Check sheet for the drawn part. Datum: minimum x, y, z corner. Units: mm. A direction names the side the tool comes from. Coordinates: 2 decimals unless noted, no trailing zeros. Write each loop counter-clockwise with the first axis right and the second up, starting at its lowest first coordinate (ties: lowest second). Pieces come first, ordered by that corner, then holes. Notation, with made-up numbers: M -0.75,61.5 L 53.25,61.5 A16 ccw 53.25,82.5 Z; hole C 61.5,60.25 d8. An arc over 180 degrees is marked long. Answer as CSV lines item,"result".
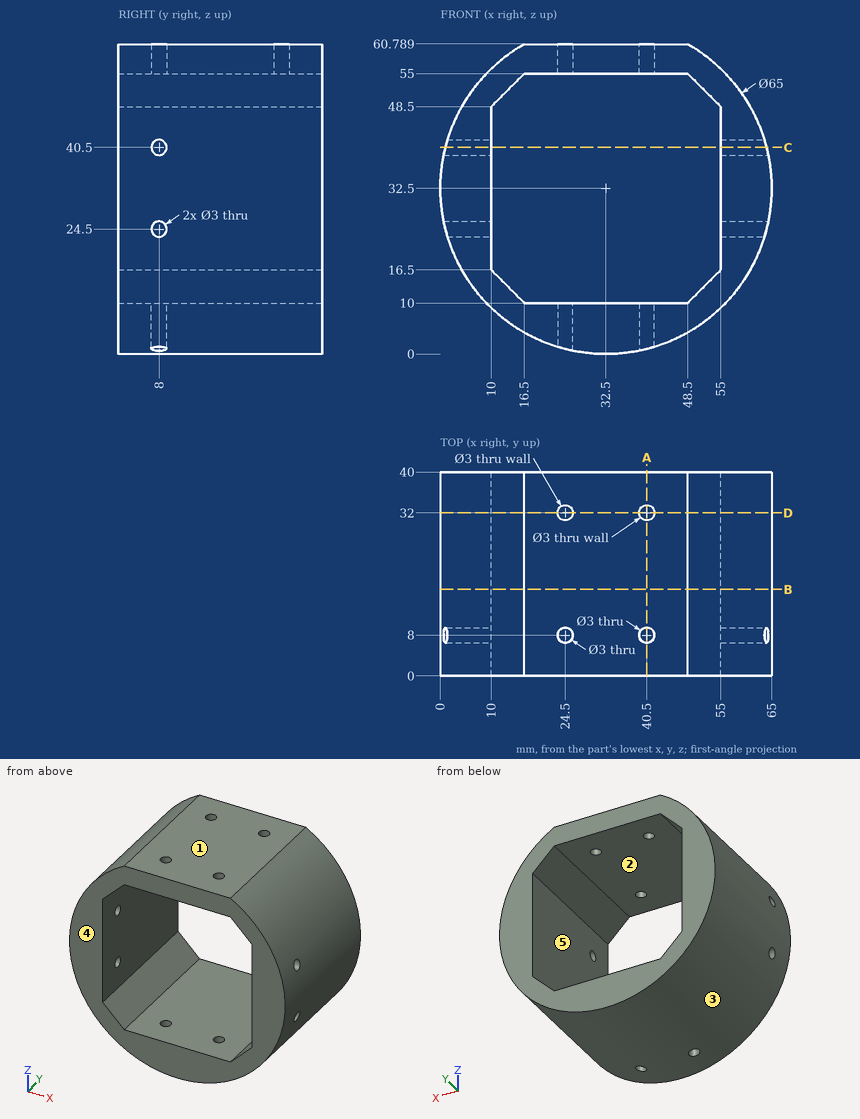
1) Section check C-C, the plane z = 40.5. Record the boundary of the cut face in (x, y), plus the area to 3 significant figures.
Answer key:
outline,"M 1,0 L 10,0 L 10,6.5 L 1,6.5 Z; M 1,9.5 L 10,9.5 L 10,40 L 1,40 Z; M 55,0 L 64,0 L 64,6.5 L 55,6.5 Z; M 55,9.5 L 64,9.5 L 64,40 L 55,40 Z"
area,"666 mm2"
2) Section check D-D, the plane y = 32. Record the boundary of the cut face in (x, z).
Answer key:
outline,"M 10,16.5 L 10,48.5 L 16.5,55 L 23,55 L 23,60.79 L 16.5,60.79 A32.5 ccw long 48.5,60.79 L 42,60.79 L 42,55 L 48.5,55 L 55,48.5 L 55,16.5 L 48.5,10 L 16.5,10 Z; M 26,55 L 39,55 L 39,60.79 L 26,60.79 Z"
3) Thickness scan on line 1 along Z through (x, y) = (41, 18); line 2 along Y through (x, z) = (5, 24) (1 decimal); line 3 along X through (y, z) = (4.5, 42.5). Record the ranges inside material, lowest first.
Answer key:
line 1,"z = 1.13 to 10, 55 to 60.79"
line 2,"y = 0 to 6.6, 9.4 to 40"
line 3,"x = 1.58 to 10, 55 to 63.42"
4) Depth check by flat-ended pin: P1, Ø1.5, axis at x = 52.5, y = 25, coming from the +Z side (1 decimal); P2, Ø4, axis at x = 24.5, y = 8, coming from the -Z side; P3, Ø16, axis at y = 19.5, z = 28.5, coming from the -X side; P4, Ø2.5, axis at y = 8, z = 24.5, coming from the -X side. Enter the tip coordinate at first touch or a pass-through.
Answer key:
P1,"stops at z = 58.7"
P2,"stops at z = 0.56"
P3,"stops at x = 0"
P4,"passes through"
5) Tool access check on the marked faces 4 and 5. Record the directions out of +Z, -Z, +X, -X, +Y, -Y that give a thin tool (end or side, any length) a straight path to the whole face; none if there is none.
Answer key:
face 4,"+Z, -Z, +X, -X, -Y"
face 5,"+Y, -Y"
6) Section check B-B, the plane y = 17. Record the boundary of the cut face in (x, z).
Answer key:
outline,"M 16.5,60.79 A32.5 ccw long 48.5,60.79 Z; hole M 10,16.5 L 16.5,10 L 48.5,10 L 55,16.5 L 55,48.5 L 48.5,55 L 16.5,55 L 10,48.5 Z"
7) Section check A-A, the plane x = 40.5. Record the boundary of the cut face in (y, z).
Answer key:
outline,"M 0,1 L 6.5,1 L 6.5,10 L 0,10 Z; M 0,55 L 6.5,55 L 6.5,60.79 L 0,60.79 Z; M 9.5,1 L 40,1 L 40,10 L 9.5,10 Z; M 9.5,55 L 30.5,55 L 30.5,60.79 L 9.5,60.79 Z; M 33.5,55 L 40,55 L 40,60.79 L 33.5,60.79 Z"
8) Mould release check, pull along Z, two halves, no side actions. Record for the marked faces 1, 2 and 3: pulls with the +Z half, pulls with the -Z half, needs draft (parallel to the pull), parting line crosses it, or undercut.
Answer key:
face 1,"pulls with the +Z half"
face 2,"undercut"
face 3,"parting line crosses it"
